Can you work these out from the model? Positions are in its coordinate system, mm. Face numbers are marked on the shaded views. A direction names the side the tool comes from. Give positions to 0.01 mm unless a question says otherwise; leave off trailing zeros. Loops run counter-clockwise (first coordinate to the right, second up) from the corner with the lowest first, then second, coordinate; pieces in that order, holes last. Notation, with made-up numbers: (45, 74) - (91, 74) arc R28 cw to (91, 105) - close; hole circle Ø1 at (51, -35.5). An arc over 180 degrees is marked (long way). Answer as a JSON object with one key per item and string values. Group by question number.
Item 1: Suppose I cut it at C-C on z = 8. Write out the boundary of the cut face in (x, y), and give its area (3 significant figures).
Item 2: Suppose I cut it at D-D on y = 5.5. Write out the boundary of the cut face in (x, z).
Item 3: Will these pins go through, and if not, where does the flat tip stop? pin 1 (5.5 mm diameter, centred on x = 13, z = 4.74, fed in from +Y); pin 2 (4 mm diameter, centred on x = 21, y = 7.5, fed in from +Z); pin 3 (4 mm diameter, centred on x = 22.5, y = 5.5, fed in from -Z); pin 4 (1 mm diameter, centred on x = 23.5, y = 12.5, fed in from +Z).
Item 4: Suppose I cut it at B-B on x = 14. Write out the boundary of the cut face in (y, z).
Item 5: Which directions (+Z, -Z, +X, -X, +Y, -Y) give clear straight access to the entire face, cutting with the end or side of a thin tool? Please do the marked faces 1, 2, 3, 4 and 5.
Item 6: Thinking about a two-plate mould opening in Y: for the marked faces 6, 7 and 8, which applies, pulls with the +Y half, pulls with the -Y half, needs draft (parallel to the pull), parting line crosses it, or undercut?
Item 7: Please list where these lines run through material, in increasing order: L1, parallel to X at y = -5.5, z = -15.35; L2, parallel to Z at x = 5.75, y = 7.75; L3, parallel to Y at x = 22.75, z = 8.5.
Item 8: Suppose I cut it at A-A on y = 1.25. Write out the boundary of the cut face in (x, z), and give its area (3 significant figures).
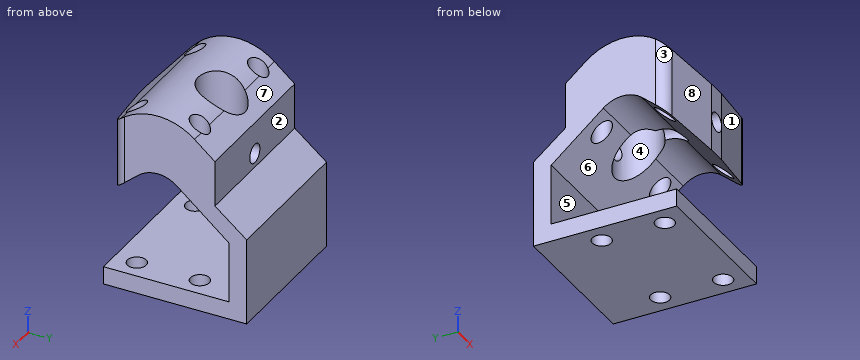
from build123d import *
from OCP.BRepFilletAPI import BRepFilletAPI_MakeChamfer

# Parameters (mm, degrees)
EXTRUDE_1_DEPTH     = 26
SKETCH_2_R          = 1.65
CUT_EXTRUDE_1_DEPTH = 45.819078563
SKETCH_3_W          = 28.1444964
SKETCH_3_H          = 6.1
CUT_EXTRUDE_2_DEPTH = 35.940261345
CUT_EXTRUDE_4_REACH = 46.819
SKETCH_5_R          = 4.1
SKETCH_6_R          = 1.65
CUT_EXTRUDE_5_DEPTH = 41.050210522
CHAMFER_1_SIZE      = 2
CHAMFER_1_SIZE2     = 11.342563639
FILLET_1_R          = 2


with BuildPart() as part:
    # 草图1 → 凸台-拉伸1 (new body)
    with BuildSketch(Plane(origin=(0, 0, 0), x_dir=(0, 0, -1), z_dir=(1, 0, 0))):
        with BuildLine():
            Line((17.407451211, 15.55), (2.245544981, 15.55))
            Line((2.245544981, 15.55), (-2.273793452, 10))
            Line((-2.273793452, 10), (-10.273793452, 10))
            Line((-10.273793452, 10), (-13.270509165, 6.44212097))
            ThreePointArc((-13.270509165, 6.44212097), (-15.622040206, 0), (-13.270509165, -6.44212097))
            Line((-13.270509165, -6.44212097), (-10.273793452, -10))
            Line((-10.273793452, -10), (-2.273793452, -10))
            Line((-2.273793452, -10), (2.245544981, -15.55))
            Line((2.245544981, -15.55), (17.407451211, -15.55))
            Line((17.407451211, -15.55), (17.407451211, 15.55))
        make_face()
        with BuildLine():
            Line((3.687588487, 12.45), (14.307451211, 12.45))
            Line((14.307451211, 12.45), (14.307451211, -12.45))
            Line((14.307451211, -12.45), (3.687588487, -12.45))
            Line((3.687588487, -12.45), (-3.977203858, -3.349902904))
            ThreePointArc((-3.977203858, -3.349902904), (-5.2, 0), (-3.977203858, 3.349902904))
            Line((-3.977203858, 3.349902904), (3.687588487, 12.45))
        make_face(mode=Mode.SUBTRACT)
    extrude(amount=EXTRUDE_1_DEPTH)

    # 草图2 → 切除-拉伸1 (cut, through all)
    with BuildSketch(Plane(origin=(0, 0, -17.407451211), x_dir=(-1, 0, 0), z_dir=(0, 0, -1))):
        with Locations((-22.5, 5.5)):
            Circle(SKETCH_2_R)
        with Locations(Location((-22.5, -5.5, 0), (0, 0, 325.181239638))):
            Circle(SKETCH_2_R)
        with Locations(Location((-3.5, -5.5, 0), (0, 0, 325.181239638))):
            Circle(SKETCH_2_R)
        with Locations(Location((-3.5, 5.5, 0), (0, 0, 180))):
            Circle(SKETCH_2_R)
    extrude(amount=-CUT_EXTRUDE_1_DEPTH, mode=Mode.SUBTRACT)

    # 草图3 → 切除-拉伸2 (cut, through all)
    with BuildSketch(Plane.ZY):
        with Locations((-3.335203011, -12.5)):
            Rectangle(SKETCH_3_W, SKETCH_3_H)
    extrude(amount=-CUT_EXTRUDE_2_DEPTH, mode=Mode.SUBTRACT)

    # 草图5 → 切除-拉伸4 (cut, up to next)
    with BuildSketch(Plane.XY.offset(15.622040206), mode=Mode.PRIVATE) as cut_extrude_4_sk1:
        with Locations(Location((13, 4.2, 0), (0, 0, 348.033440949))):
            Circle(SKETCH_5_R)
    cut_extrude_4_tool1 = extrude(cut_extrude_4_sk1.sketch, amount=-CUT_EXTRUDE_4_REACH, mode=Mode.PRIVATE) & part.part
    add(cut_extrude_4_tool1.solids().sort_by_distance((13, 4.2, 15.62204))[0], mode=Mode.SUBTRACT)

    # 草图6 → 切除-拉伸5 (cut, through all)
    with BuildSketch(Plane.XZ.offset(9.45)):
        with Locations(Location((13, 4.737045189, 0), (0, 0, 270))):
            Circle(SKETCH_6_R)
    extrude(amount=-CUT_EXTRUDE_5_DEPTH, mode=Mode.SUBTRACT)

    # 倒角1: one chamfer whose edges measure the first distance from different faces: ONE call of the kernel's chamfer builder (chamfer() names one face for all edges)
    chamfer_1_edges_1 = [part.edges().sort_by_distance(p)[0] for p in [
        (0, -9.45, 4.78814218),
    ]]
    chamfer_1_side_1 = [part.faces().sort_by_distance(p)[0] for p in [
        (0, -9.035760057, -15.857451211),
    ]]
    chamfer_1_edges_2 = [part.edges().sort_by_distance(p)[0] for p in [
        (26, -9.45, 4.78814218),
    ]]
    chamfer_1_side_2 = [part.faces().sort_by_distance(p)[0] for p in [
        (26, -9.035760057, -15.857451211),
    ]]
    chamfer_1 = BRepFilletAPI_MakeChamfer(part.part.solid().wrapped)
    for e in chamfer_1_edges_1:
        chamfer_1.Add(CHAMFER_1_SIZE, CHAMFER_1_SIZE2, e.wrapped, chamfer_1_side_1[0].wrapped)  # the first distance lies on this face
    for e in chamfer_1_edges_2:
        chamfer_1.Add(CHAMFER_1_SIZE, CHAMFER_1_SIZE2, e.wrapped, chamfer_1_side_2[0].wrapped)  # the first distance lies on this face
    add(Compound.cast(chamfer_1.Shape()), mode=Mode.REPLACE)

    # 圆角1
    # the kernel refuses this fillet: 2 mm, written as the material it takes off along each edge
    with BuildSketch(Plane(origin=(26, -7.45, -3.671707212), x_dir=(-0.9848077530122086, -0.17364817766692747, 0), z_dir=(0, 0, 1))) as fillet_1_piece_1:
        with BuildLine():
            CenterArc((FILLET_1_R * 0.839099631177, -FILLET_1_R), FILLET_1_R, 90, 80)
            Line((-FILLET_1_R * 0.145708121835, -FILLET_1_R * 0.826351822333), (0, 0))
            Line((0, 0), (FILLET_1_R * 0.839099631177, 0))
        make_face()
    extrude(amount=20.288802329, mode=Mode.SUBTRACT)
    with BuildSketch(Plane(origin=(0, -7.45, 16.617095117), x_dir=(0, 1, 0), z_dir=(0, 0, -1))) as fillet_1_piece_2:
        with BuildLine():
            CenterArc((FILLET_1_R * 0.839099631177, FILLET_1_R), FILLET_1_R, 190, 80)
            Line((-FILLET_1_R * 0.145708121835, FILLET_1_R * 0.826351822333), (0, 0))
            Line((0, 0), (FILLET_1_R * 0.839099631177, 0))
        make_face()
    extrude(amount=20.288802329, mode=Mode.SUBTRACT)


solid = part.part
Worked out:
{
 "1": {"outline": "(0, -5.77) arc R2 ccw to (1.65, -7.74) - (11.34, -9.45) - (14.66, -9.45) - (24.35, -7.74) arc R2 ccw to (26, -5.77) - (26, 10) - (0, 10) - close; hole circle Ø3.3 at (3.5, -5.5); hole circle Ø3.3 at (3.5, 5.5); hole circle Ø8.2 at (13, 4.2); hole circle Ø3.3 at (22.5, -5.5); hole circle Ø3.3 at (22.5, 5.5)", "area": "395 mm2"},
 "2": {"outline": "(0, -17.41) - (1.85, -17.41) - (1.85, -14.31) - (0, -14.31) - close; (0, 2.17) - (1.85, 2.17) - (1.85, 13.97) - (0, 13.97) - close; (5.15, -17.41) - (20.85, -17.41) - (20.85, -14.31) - (5.15, -14.31) - close; (5.15, 2.17) - (9.11, 2.17) - (9.11, 13.97) - (5.15, 13.97) - close; (16.89, 2.17) - (20.85, 2.17) - (20.85, 13.97) - (16.89, 13.97) - close; (24.15, -17.41) - (26, -17.41) - (26, -14.31) - (24.15, -14.31) - close; (24.15, 2.17) - (26, 2.17) - (26, 13.97) - (24.15, 13.97) - close"},
 "3": {"pin 1": "stops at y = 10.35", "pin 2": "stops at z = 13.97", "pin 3": "stops at z = -17.41", "pin 4": "stops at z = 0.65"},
 "4": {"outline": "(-9.45, -17.41) - (15.55, -17.41) - (15.55, -2.25) - (10, 2.27) - (10, 3.42) - (8.18, 3.42) - (8.18, -0.09) - (12.45, -3.69) - (12.45, -14.31) - (-9.45, -14.31) - close; (-9.45, -1.16) - (-4.01, 3.42) - (-9.45, 3.42) - close; (-9.45, 6.05) - (0.22, 6.05) - (0.22, 15.62) arc R10 ccw to (-6.44, 13.27) - (-9.45, 10.74) - close; (8.18, 6.05) - (10, 6.05) - (10, 10.27) - (8.18, 11.81) - close"},
 "5": {"face 1": "+Z, +X, -Y", "face 2": "+Z, +X, -X, +Y", "face 3": "+Z, -X, -Y", "face 4": "+Z", "face 5": "+X, -X, -Y"},
 "6": {"face 6": "undercut", "face 7": "pulls with the +Y half", "face 8": "pulls with the -Y half"},
 "7": {"L1": "x = 0 to 1.85, 5.15 to 20.85, 24.15 to 26", "L2": "z = -17.41 to -14.31, 0.27 to 12.17", "L3": "y = -8.02 to -7.13, -3.87 to 3.87, 7.13 to 10"},
 "8": {"outline": "(0, -17.41) - (26, -17.41) - (26, -14.31) - (0, -14.31) - close; (0, 5.05) - (10.15, 5.05) - (10.15, 15.54) - (0, 15.54) - close; (15.85, 5.05) - (26, 5.05) - (26, 15.54) - (15.85, 15.54) - close", "area": "294 mm2"}
}
